Here's how the part is built. I have some questions about the finished solid (model axes, mm). Give positions to 0.01 mm unless a question says otherwise; leave off trailing zeros. Loops run counter-clockwise (first coordinate to the right, second up) from the corner with the lowest first, then second, coordinate; pieces in that order, holes last. Notation, with made-up numbers: (8.5, 39.25) - (31.5, 39.25) arc R30 ccw to (31.5, 66.25) - close; hole circle Ø8 at (41.5, 49.25). An arc over 180 degrees is marked (long way). One line per item, written item: value. Start each with the question number.
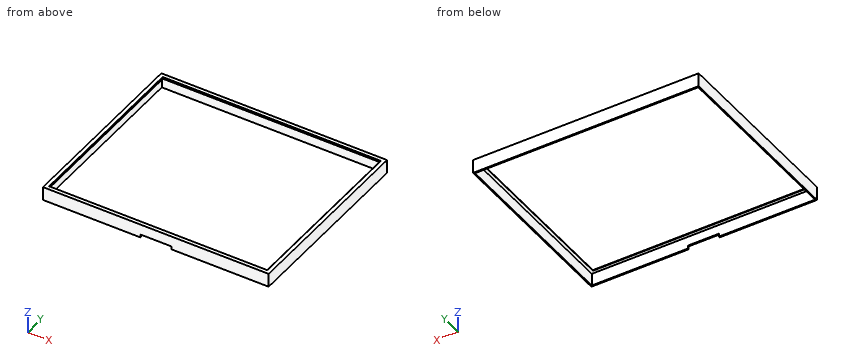
```python
from build123d import *

# Parameters (mm, degrees)
F0_W     = 363
F0_H     = 301
F0_W_2   = 359
F0_H_2   = 297
F0_W_3   = 349
F0_H_3   = 287
F1_DEPTH = 22
F2_DEPTH = 25
F3_DEPTH = 20
F4_SIZE  = 1
F5_W     = 50
F5_H     = 5
F6_DEPTH = 25


with BuildPart() as f1:
    # F0 (on Top) → F1 (new body)
    with BuildSketch(Plane.XY):
        Rectangle(F0_W, F0_H)
        Rectangle(F0_W_2, F0_H_2, mode=Mode.SUBTRACT)
        Rectangle(F0_W_3, F0_H_3)
        Rectangle(F0_W_2, F0_H_2)
        Rectangle(F0_W_3, F0_H_3, mode=Mode.SUBTRACT)
    extrude(amount=F1_DEPTH)

    # F0 (on Top) → F2 (cut)
    with BuildSketch(Plane.XY):
        Rectangle(F0_W_3, F0_H_3)
    extrude(amount=F2_DEPTH, mode=Mode.SUBTRACT)

    # F0 (on Top) → F3 (cut)
    with BuildSketch(Plane.XY):
        Rectangle(F0_W_2, F0_H_2)
        Rectangle(F0_W_3, F0_H_3, mode=Mode.SUBTRACT)
    extrude(amount=F3_DEPTH, mode=Mode.SUBTRACT)

    # F4
    f4_edges = [f1.edges().sort_by_distance(p)[0] for p in [
        (0, -143.5, 22),
        (-174.5, 0, 22),
        (0, 143.5, 22),
        (174.5, 0, 22),
    ]]
    chamfer(f4_edges, length=F4_SIZE)

    # F5 (on face) → F6 (cut)
    with BuildSketch(Plane.XZ.offset(150.5)):
        with Locations((0, 2.5)):
            Rectangle(F5_W, F5_H)
    extrude(amount=-F6_DEPTH, mode=Mode.SUBTRACT)


solid = f1.part
```
(1) If we section it at C-C on z = 12.25: List the corners of the cut face in (x, y) for me, plus the area to 3 significant figures.
(2) If we section it at B-B on y = 108: List the corners of the cut face in (x, z) for me.
(3) Please list where these lines run through material, in increasing order: probe 1 along X at (y, z) = (83, 11); probe 2 along Y at (x, z) = (54.5, 16.5). Write a range as from..to.
(4) Will this pin go through, and if not, where does the flat tip stop? pin 1 (1.6 mm diameter, centred on x = -4, y = -149.5, fed in from -Z).
(5) If we section it at A-A on x = -90: List the corners of the cut face in (y, z) for me, plus the area to 3 significant figures.
Found:
1. outline: (-181.5, -150.5) - (181.5, -150.5) - (181.5, 150.5) - (-181.5, 150.5) - close; hole (-179.5, -148.5) - (179.5, -148.5) - (179.5, 148.5) - (-179.5, 148.5) - close
1. area: 2,640 mm^2
2. outline: (-181.5, 0) - (-179.5, 0) - (-179.5, 20) - (-174.5, 20) - (-174.5, 21) - (-175.5, 22) - (-181.5, 22) - close; (174.5, 20) - (179.5, 20) - (179.5, 0) - (181.5, 0) - (181.5, 22) - (175.5, 22) - (174.5, 21) - close
3. probe 1: -181.5..-179.5, 179.5..181.5
3. probe 2: -150.5..-148.5, 148.5..150.5
4. pin 1: z = 5
5. outline: (-150.5, 0) - (-148.5, 0) - (-148.5, 20) - (-143.5, 20) - (-143.5, 21) - (-144.5, 22) - (-150.5, 22) - close; (143.5, 20) - (148.5, 20) - (148.5, 0) - (150.5, 0) - (150.5, 22) - (144.5, 22) - (143.5, 21) - close
5. area: 107 mm^2
